```python
from build123d import *

# Parameters (mm, degrees)
SKETCH1_R               = 4.55
SKETCH1_R_2             = 1.55
BOSS_EXTRUDE1_DEPTH     = 9.1
SKETCH2_R               = 1.55
BOSS_EXTRUDE2_DEPTH     = 3
SKETCH3_W               = 15.1
SKETCH3_H               = 9.1
BOSS_EXTRUDE3_DEPTH     = 3
CUT_EXTRUDE1_REACH      = 26.036
CUT_EXTRUDE1_END_RADIUS = 3.55
SKETCH4_R               = 1.55
SKETCH5_R               = 1.55
CUT_EXTRUDE2_DEPTH      = 2.5
CHAMFER1_SIZE           = 1
CHAMFER2_SIZE           = 3


with BuildPart() as part:
    # Sketch1 → Boss-Extrude1 (new body)
    # profile 1 of 3: a face of its own
    with BuildSketch(Plane.XY):
        with Locations((-94.564189657, 2.5)):
            Circle(SKETCH1_R)
        with Locations((-94.564189657, 2.5)):
            Circle(SKETCH1_R_2, mode=Mode.SUBTRACT)
    # profile 2 of 3: a face of its own
    with BuildSketch(Plane.XY):
        with BuildLine():
            ThreePointArc((-94.564189657, -2.05), (-99.114189657, 2.5), (-94.564189657, 7.05))
            Line((-94.564189657, 7.05), (-100.114189657, 7.05))
            Line((-100.114189657, 7.05), (-100.114189657, -2.05))
            Line((-100.114189657, -2.05), (-94.564189657, -2.05))
        make_face()
    # profile 3 of 3: a face of its own
    with BuildSketch(Plane.XY):
        with BuildLine():
            Line((-85.014189657, 7.05), (-94.564189657, 7.05))
            ThreePointArc((-94.564189657, 7.05), (-91.346853802, 5.717335854), (-90.014189657, 2.5))
            ThreePointArc((-90.014189657, 2.5), (-91.346853802, -0.717335854), (-94.564189657, -2.05))
            Line((-94.564189657, -2.05), (-85.014189657, -2.05))
            Line((-85.014189657, -2.05), (-85.014189657, 7.05))
        make_face()
    extrude(amount=BOSS_EXTRUDE1_DEPTH)



with BuildPart() as body_2:
    # Sketch2 → Boss-Extrude2 (new body)
    # profile 1 of 2: a face of its own
    with BuildSketch(Plane(origin=(0, 0, -3), x_dir=(-1, 0, 0), z_dir=(0, 0, -1))):
        with BuildLine():
            ThreePointArc((95.352918097, 6.981116764), (94.960054991, 7.032746478), (94.564189657, 7.05))
            ThreePointArc((94.564189657, 7.05), (90.014189657, 2.5), (94.564189657, -2.05))
            ThreePointArc((94.564189657, -2.05), (94.960054991, -2.032746478), (95.352918097, -1.981116763))
            ThreePointArc((95.352918097, -1.981116763), (98.049244492, -0.42521671), (99.114189657, 2.5))
            ThreePointArc((99.114189657, 2.5), (98.049244492, 5.42521671), (95.352918097, 6.981116764))
        make_face()
        with Locations(Location((94.564189657, 2.5, 0), (0, 0, 180))):
            Circle(SKETCH2_R, mode=Mode.SUBTRACT)
    # profile 2 of 2: a face of its own
    with BuildSketch(Plane(origin=(0, 0, -3), x_dir=(-1, 0, 0), z_dir=(0, 0, -1))):
        with BuildLine():
            Line((100.114189657, -2.05), (100.114189657, 7.05))
            Line((100.114189657, 7.05), (94.96156182, 7.05))
            Line((94.96156182, 7.05), (95.352918097, 6.981116764))
            ThreePointArc((95.352918097, 6.981116764), (98.049244492, 5.42521671), (99.114189657, 2.5))
            ThreePointArc((99.114189657, 2.5), (98.049244492, -0.42521671), (95.352918097, -1.981116763))
            Line((95.352918097, -1.981116763), (94.96156182, -2.05))
            Line((94.96156182, -2.05), (100.114189657, -2.05))
        make_face()
    extrude(amount=BOSS_EXTRUDE2_DEPTH)


with BuildPart() as part_1:
    add(part.part)

    add(body_2.part)  # Boss-Extrude3 merges body 2
    # Sketch3 → Boss-Extrude3 (add)
    with BuildSketch(Plane.ZY.offset(100.114189657)):
        with Locations((1.55, 2.5)):
            Rectangle(SKETCH3_W, SKETCH3_H)
    extrude(amount=BOSS_EXTRUDE3_DEPTH)

    # Loft1: read off the stored shape, not the designer's step
    # Loft1: loft between two sections, ruled curve by curve
    loft1_from = [
        Edge.make_bspline([(-85.014189657, -2.05, 9.1), (-85.014189657, -2.05, 8.341666667), (-85.014189657, -2.05, 7.583333333), (-85.014189657, -2.05, 6.066666667), (-85.014189657, -2.05, 5.308333333), (-85.014189657, -2.05, 3.791666667), (-85.014189657, -2.05, 3.033333333), (-85.014189657, -2.05, 1.516666667), (-85.014189657, -2.05, 0.758333333), (-85.014189657, -2.05, 0)], [0, 0, 0, 0, 0.25, 0.25, 0.5, 0.5, 0.75, 0.75, 1, 1, 1, 1], 3),
        Edge.make_bspline([(-85.014189657, -2.05, 0), (-85.014189657, -1.291666667, 0), (-85.014189657, -0.533333333, 0), (-85.014189657, 0.983333333, 0), (-85.014189657, 1.741666667, 0), (-85.014189657, 3.258333333, 0), (-85.014189657, 4.016666667, 0), (-85.014189657, 5.533333333, 0), (-85.014189657, 6.291666667, 0), (-85.014189657, 7.05, 0)], [0, 0, 0, 0, 0.25, 0.25, 0.5, 0.5, 0.75, 0.75, 1, 1, 1, 1], 3),
        Edge.make_bspline([(-85.014189657, 7.05, 9.1), (-85.014189657, 6.291666667, 9.1), (-85.014189657, 5.533333333, 9.1), (-85.014189657, 4.016666667, 9.1), (-85.014189657, 3.258333333, 9.1), (-85.014189657, 1.741666667, 9.1), (-85.014189657, 0.983333333, 9.1), (-85.014189657, -0.533333333, 9.1), (-85.014189657, -1.291666667, 9.1), (-85.014189657, -2.05, 9.1)], [0, 0, 0, 0, 0.25, 0.25, 0.5, 0.5, 0.75, 0.75, 1, 1, 1, 1], 3),
        Edge.make_bspline([(-85.014189657, 7.05, 0), (-85.014189657, 7.05, 0.758333333), (-85.014189657, 7.05, 1.516666667), (-85.014189657, 7.05, 3.033333333), (-85.014189657, 7.05, 3.791666667), (-85.014189657, 7.05, 5.308333333), (-85.014189657, 7.05, 6.066666667), (-85.014189657, 7.05, 7.583333333), (-85.014189657, 7.05, 8.341666667), (-85.014189657, 7.05, 9.1)], [0, 0, 0, 0, 0.25, 0.25, 0.5, 0.5, 0.75, 0.75, 1, 1, 1, 1], 3),
    ]
    loft1_to = [
        Edge.make_bspline([(-82.014189657, 0.378679656, 6.671320344), (-82.014189657, 0.128679656, 6.421320344), (-82.014189657, -0.095475789, 6.106038327), (-82.014189657, -0.410975479, 5.377025758), (-82.014189657, -0.5, 4.964213562), (-82.014189657, -0.5, 4.135786438), (-82.014189657, -0.410975479, 3.722974242), (-82.014189657, -0.095475789, 2.993961673), (-82.014189657, 0.128679656, 2.678679656), (-82.014189657, 0.378679656, 2.428679656)], [0, 0, 0, 0, 0.25, 0.25, 0.5, 0.5, 0.75, 0.75, 1, 1, 1, 1], 3),
        Edge.make_bspline([(-82.014189657, 0.378679656, 2.428679656), (-82.014189657, 0.628679656, 2.178679656), (-82.014189657, 0.943961673, 1.954524211), (-82.014189657, 1.672974242, 1.639024521), (-82.014189657, 2.085786438, 1.55), (-82.014189657, 2.914213562, 1.55), (-82.014189657, 3.327025758, 1.639024521), (-82.014189657, 4.056038327, 1.954524211), (-82.014189657, 4.371320344, 2.178679656), (-82.014189657, 4.621320344, 2.428679656)], [0, 0, 0, 0, 0.25, 0.25, 0.5, 0.5, 0.75, 0.75, 1, 1, 1, 1], 3),
        Edge.make_bspline([(-82.014189657, 4.621320344, 6.671320344), (-82.014189657, 4.371320344, 6.921320344), (-82.014189657, 4.056038327, 7.145475789), (-82.014189657, 3.327025758, 7.460975479), (-82.014189657, 2.914213562, 7.55), (-82.014189657, 2.085786438, 7.55), (-82.014189657, 1.672974242, 7.460975479), (-82.014189657, 0.943961673, 7.145475789), (-82.014189657, 0.628679656, 6.921320344), (-82.014189657, 0.378679656, 6.671320344)], [0, 0, 0, 0, 0.25, 0.25, 0.5, 0.5, 0.75, 0.75, 1, 1, 1, 1], 3),
        Edge.make_bspline([(-82.014189657, 4.621320344, 2.428679656), (-82.014189657, 4.871320344, 2.678679656), (-82.014189657, 5.095475789, 2.993961673), (-82.014189657, 5.410975479, 3.722974242), (-82.014189657, 5.5, 4.135786438), (-82.014189657, 5.5, 4.964213562), (-82.014189657, 5.410975479, 5.377025758), (-82.014189657, 5.095475789, 6.106038327), (-82.014189657, 4.871320344, 6.421320344), (-82.014189657, 4.621320344, 6.671320344)], [0, 0, 0, 0, 0.25, 0.25, 0.5, 0.5, 0.75, 0.75, 1, 1, 1, 1], 3),
    ]
    loft1 = Solid(Shell([*[Face.make_surface_from_curves(loft1_from[k], loft1_to[k]) for k in range(4)], Face(Wire(loft1_from)), Face(Wire(loft1_to))]))
    add(loft1)

    # Cut-Extrude1: up to this cylinder (the profile starts outside it)
    cut_extrude1_end = Plane(origin=(-94.564189657, 2.5, 4.55), z_dir=(0, 0, -1)) * Cylinder(CUT_EXTRUDE1_END_RADIUS, 60.172, mode=Mode.PRIVATE)
    # Sketch4 → Cut-Extrude1 (cut, up to the surface)
    with BuildSketch(Plane(origin=(-82.014189657, 0, 0), x_dir=(0, 0, -1), z_dir=(1, 0, 0)), mode=Mode.PRIVATE) as cut_extrude1_sk1:
        with Locations((-4.55, 2.5)):
            Circle(SKETCH4_R)
    cut_extrude1_tool1 = extrude(cut_extrude1_sk1.sketch, amount=-CUT_EXTRUDE1_REACH, mode=Mode.PRIVATE) - cut_extrude1_end
    add(cut_extrude1_tool1.solids().sort_by_distance((-82.01419, 2.5, 4.55))[0], mode=Mode.SUBTRACT)

    # Sketch5 → Cut-Extrude2 (cut)
    # profile 1 of 2: a face of its own
    with BuildSketch(Plane.ZY.offset(87.014189657)):
        Polygon((4.55, 5.675426481), (7.3, 4.08771324), (7.3, 7.05), (1.8, 7.05), (1.8, 4.08771324), align=None)
    # profile 2 of 2: a face of its own
    with BuildSketch(Plane.ZY.offset(87.014189657)):
        Polygon((7.3, 0.91228676), (7.3, 4.08771324), (4.55, 5.675426481), (1.8, 4.08771324), (1.8, 0.91228676), (4.55, -0.675426481), align=None)
        with Locations(Location((4.55, 2.5, 0), (0, 0, 180))):
            Circle(SKETCH5_R, mode=Mode.SUBTRACT)
    extrude(amount=CUT_EXTRUDE2_DEPTH, mode=Mode.SUBTRACT)

    # Chamfer1
    chamfer1_edges = [part_1.edges().sort_by_distance(p)[0] for p in [
        (-87.014189657, 7.05, 4.55),
        (-88.264189657, 7.05, 7.3),
        (-88.264189657, 7.05, 1.8),
        (-89.514189657, 7.05, 4.55),
    ]]
    chamfer(chamfer1_edges, length=CHAMFER1_SIZE)

    # Chamfer2
    chamfer2_edges = [part_1.edges().sort_by_distance(p)[0] for p in [
        (-103.114189657, 2.5, 9.1),
    ]]
    chamfer(chamfer2_edges, length=CHAMFER2_SIZE)


solid = part_1.part
```
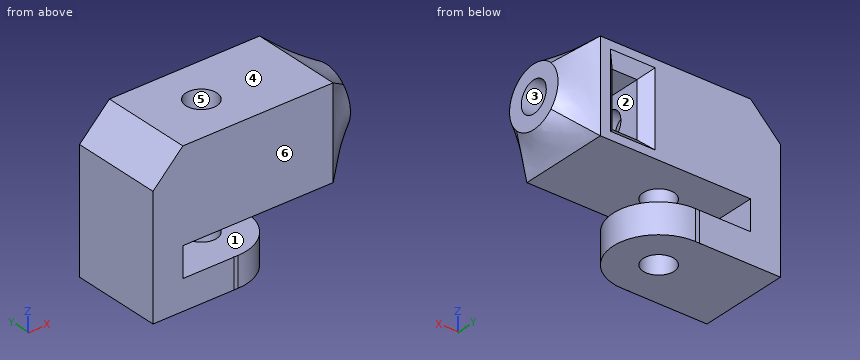
The listing builds one solid part. Answer for the finished solid, in the listing's coordinates (mm). Face numbers are marked on the shaded views. A direction names the side the tool comes from. Give positions to 0.01 mm unless a question says otherwise; leave off trailing zeros. Loops run counter-clockwise (first coordinate to the right, second up) from the corner with the lowest first, then second, coordinate; pieces in that order, holes last. Notation, with made-up numbers: M 31,77 L 38,77 A22 cw 38,108 Z; hole C 78.5,87 d7. An arc over 180 degrees is marked long. One line per item, written item: value.
Q1. Determine the mould class of the marked faces 4, 5 and 6 for opening direction Y: +Y half, -Y half, draft (parallel to the pull), parting line (faces both ways), or undercut.
Working result:
face 4: draft
face 5: undercut
face 6: -Y half
Q2. A cutting plane is placed at D-D on x = -93.25. Determine the outline of the cut face in (y, z).
Working result:
outline: M -2.05,0 L 1.68,0 L 1.68,9.1 L -2.05,9.1 Z; M -1.86,-6 L 1.68,-6 L 1.68,-3 L -1.86,-3 Z; M 3.32,-6 L 6.86,-6 L 6.86,-3 L 3.32,-3 Z; M 3.32,0 L 7.05,0 L 7.05,9.1 L 3.32,9.1 Z
Q3. Flat-ended cylindrical pins translate along their axes: P1, Ø3.5, axis at y = 2, z = -1, coming from the +X side; P2, Ø1.2, axis at x = -88.5, y = 3, coming from the -Z side. Find the tip coordinate at first contact, or state that the pin passes through.
Working result:
P1: stops at x = -83.58
P2: stops at z = 0
Q4. A cutting plane is placed at C-C on y = 2.5. Give the number of separate pieces and of enclosed holes in the cut face, then the cut area to 3 significant figures.
Working result:
separate pieces: 3
enclosed holes: 0
area: 160 mm^2
Q5. A cutting plane is placed at B-B on z = -3.25. Determine the outline of the cut face in (x, y), then the cut area to 3 significant figures.
Working result:
outline: M -103.11,-2.05 L -94.96,-2.05 L -95.35,-1.98 A4.55 ccw long -95.35,6.98 L -94.96,7.05 L -103.11,7.05 Z; hole C -94.56,2.5 d3.1
area: 103 mm^2
Q6. For the marked faces 1, 2 and 3, determine the directions among +Z, -Z, +X, -X, +Y, -Y from which every point of the face is accessible in a straight line to the end or side of a thin tool.
Working result:
face 1: +X, +Y, -Y
face 2: +Y
face 3: +X
Q7. A cutting plane is placed at A-A on x = -98.5. Determine the outline of the cut face in (y, z), then the cut area to 3 significant figures.
Working result:
outline: M -2.05,-6 L 7.05,-6 L 7.05,-3 L -2.05,-3 Z; M -2.05,0 L 7.05,0 L 7.05,9.1 L -2.05,9.1 Z
area: 110 mm^2
Q8. Find the intervals of material crossed by line 1 (Z direction, x = -90.9, y = 2.5); line 2 (Z direction, x = -89, y = 3.25); line 3 (X direction, y = 3, z = 2), in increasing order. Write a range as from..to.
Working result:
line 1: z = -6..-3, 0..3, 6.1..9.1
line 2: z = 0..1.8, 7.3..9.1
line 3: x = -103.11..-96.03, -93.1..-89.51, -87.01..-82.01
